Autodesk Inventor part; units mm, degrees
ref_plane "YZ Plane" through (0, 0, 0) normal (1, 0, 0) x (0, 1, 0)
ref_plane "XZ Plane" through (0, 0, 0) normal (0, 1, 0) x (-1, 0, 0)
ref_plane "XY Plane" through (0, 0, 0) normal (0, 0, 1) x (1, 0, 0)
sketch "Skizze1" plane through (0, 0, 0) normal (0, 0, 1) x (1, 0, 0)
  line L0 (-39.95, 42.95) -> (-39.95, -42.95)
  line L1 (-39.95, -42.95) -> (39.95, -42.95)
  line L2 (39.95, -42.95) -> (39.95, 42.95)
  line L3 (39.95, 42.95) -> (-39.95, 42.95)
  line L4 (-36.95, 39.95) -> (-15, 39.95)
  line L5 (36.95, 39.95) -> (36.95, -39.95)
  line L6 (36.95, -39.95) -> (-36.95, -39.95)
  line L7 (-36.95, -39.95) -> (-36.95, 39.95)
  line L8 (-36.95, 39.95) -> (36.95, -39.95) construction
  line L9 (36.95, 39.95) -> (-36.95, -39.95) construction
  line L10 (0, -67.13) -> (0, 67.13)
  line L11 (-15, 39.95) -> (-15, 42.95)
  line L12 (15, 39.95) -> (15, 42.95)
  line L13 (15, 39.95) -> (36.95, 39.95)
  line L14 (44.95, -47.95) -> (-44.95, -47.95)
  line L15 (-44.95, -47.95) -> (-44.95, 47.95)
  line L16 (-44.95, 47.95) -> (-15, 47.95)
  line L17 (44.95, 47.95) -> (44.95, -47.95)
  line L18 (44.95, -47.95) -> (-44.95, 47.95) construction
  line L19 (-44.95, -47.95) -> (44.95, 47.95) construction
  line L20 (-15, 42.95) -> (-15, 47.95)
  line L21 (15, 42.95) -> (15, 47.95)
  line L22 (15, 47.95) -> (44.95, 47.95)
  point P0 (0, 0)
  point P1 (-15, 41.45)
  dimension "d0" = 3
  dimension "d1" = 3
  dimension "d2" = 30
  dimension "d4" = 5
  dimension "d5" = 5
extrude "Extrusion1" add sketch "Skizze1" along normal blind 10 contours L3 L11 L4 L7 L6 L10 L1 L0 | L0 L1 L10 L14 L15 L16 L20 L3 | L10 L6 L5 L13 L12 L3 L2 L1 | L1 L2 L3 L21 L22 L17 L14 L10
sketch "Skizze2" plane through (0, 0, 0) normal (0, 0, -1) x (-1, 0, 0)
  line L0 (-39.95, 42.95) -> (39.95, 42.95)
  line L1 (39.95, 42.95) -> (39.95, -42.95)
  line L2 (39.95, -42.95) -> (-39.95, -42.95)
  line L3 (-39.95, -42.95) -> (-39.95, 42.95)
  line L4 (-44.95, -47.95) -> (-44.95, 47.95)
  line L5 (-44.95, 47.95) -> (-15, 47.95)
  line L6 (44.95, -47.95) -> (-44.95, -47.95)
  line L7 (44.95, 47.95) -> (44.95, -47.95)
  line L8 (15, 47.95) -> (44.95, 47.95)
  line L9 (15, 39.95) -> (15, 47.95)
  line L10 (15, 47.95) -> (44.95, 47.95)
  line L11 (15, 47.95) -> (15, 42.95)
  line L12 (15, 39.95) -> (15, 47.95)
  line L13 (15, 47.95) -> (44.95, 47.95)
  line L14 (44.95, 47.95) -> (44.95, -47.95)
  line L15 (44.95, -47.95) -> (44.95, 47.95)
  line L16 (15, 42.95) -> (39.95, 42.95)
  line L17 (39.95, 42.95) -> (39.95, -42.95)
  line L18 (39.95, -42.95) -> (-39.95, -42.95)
  line L19 (-39.95, 42.95) -> (-39.95, -42.95)
  line L20 (-39.95, 42.95) -> (-15, 42.95)
  line L21 (-15, 47.95) -> (-15, 39.95)
  line L22 (-15, 42.95) -> (-15, 47.95)
  line L23 (-44.95, -47.95) -> (-44.95, 47.95)
  line L24 (-15, 47.95) -> (-44.95, 47.95)
  line L25 (-44.95, 47.95) -> (-44.95, -47.95)
  line L26 (-40.1, -43.1) -> (40.1, -43.1)
  line L27 (40.1, -43.1) -> (40.1, 43.1)
  line L28 (40.1, 43.1) -> (-40.1, 43.1)
  line L29 (-40.1, 43.1) -> (-40.1, -43.1)
  line L30 (-40.1, -43.1) -> (40.1, 43.1) construction
  line L31 (40.1, -43.1) -> (-40.1, 43.1) construction
  point P0 (0, 0)
  point P1 (15, 43.1)
  point P2 (-15, 43.1)
  dimension "d35" = 80.2
  dimension "d36" = 86.2
extrude "Extrusion2" add sketch "Skizze2" along normal blind 1.6 contours L28 L29 L26 L27 L9 L8 L7 L6 L4 L5 L21
sketch "Skizze3" plane through (0, 0, 10) normal (0, 0, 1) x (1, 0, 0)
  line L0 (44.95, -47.95) -> (-44.95, -47.95)
  line L1 (-44.95, 47.95) -> (44.95, 47.95)
  line L2 (44.95, 47.95) -> (44.95, -47.95)
  line L3 (44.95, -47.95) -> (-44.95, -47.95)
  line L4 (-44.95, -47.95) -> (-44.95, 47.95)
  point P0 (0, 0)
extrude "Extrusion3" add sketch "Skizze3" along normal blind 2
sketch "Skizze4" plane through (0, 0, 10) normal (0, 0, -1) x (-1, 0, 0)
  line L0 (15, 39.95) -> (15, 47.95)
  line L1 (-15, 47.95) -> (15, 47.95)
  line L2 (-15, 47.95) -> (-15, 39.95)
  line L3 (-15, 39.95) -> (-36.95, 39.95)
  line L4 (-36.95, 39.95) -> (-36.95, -39.95)
  line L5 (-36.95, -39.95) -> (36.95, -39.95)
  line L6 (36.95, -39.95) -> (36.95, 39.95)
  line L7 (36.95, 39.95) -> (15, 39.95)
  line L8 (0, -67.13) -> (0, 67.13)
  line L9 (-15, 47.95) -> (15, 47.95)
  line L10 (15, 47.95) -> (7.5, 47.95)
  line L11 (7.5, 47.95) -> (7.5, 44.95)
  line L12 (7.5, 44.95) -> (15, 44.95)
  line L13 (15, 44.95) -> (15, 47.95)
  line L14 (-15, 39.95) -> (-15, 47.95)
  line L15 (15, 47.95) -> (-15, 47.95)
  line L16 (-7.5, 47.95) -> (-7.5, 44.95)
  line L17 (-7.5, 44.95) -> (-15, 44.95)
  point P0 (0, 0)
  point P1 (-7.5, 47.95)
  point P2 (-15, 44.95)
  point P3 (15, 44.95)
  point P4 (7.5, 47.95)
  point P5 (7.5, 46.45)
  point P6 (11.25, 47.95)
  dimension "d14" = 15
  dimension "d15" = 3
extrude "Extrusion4" add sketch "Skizze4" along normal up to surface (11.6 mm away) contours L12 L11 L1 L0 | L16 L17 L2 L1
fillet "Rundung1" radius 2 2 edges at (-7.5, 46.45, 10) (7.5, 46.45, 10)
fillet "Rundung2" [suppressed]
fillet "Rundung3" [suppressed]
sketch "Skizze5" plane through (0, 0, 10) normal (0, 0, -1) x (-1, 0, 0)
  circle A0 centre (-26.75, 21.7) radius 1.1
  circle A1 centre (27.25, 21.65) radius 1.1
  point P0 (0, 0)
extrude "Extrusion5" cut sketch "Skizze5" against normal through all
sketch "Skizze6" plane through (0, 0, 10) normal (0, 0, -1) x (-1, 0, 0)
  point P0 (0, 0)
sketch "Skizze7" plane through (0, 0, 10) normal (0, 0, -1) x (-1, 0, 0)
  circle A0 centre (27.25, 21.65) radius 1.1
  circle A1 centre (-26.75, 21.7) radius 1.1
  line L0 (-5.5, 44.95) -> (-5.5, 47.95)
  line L1 (-5.5, 44.95) -> (-15, 44.95)
  line L2 (-15, 44.95) -> (-15, 39.95)
  line L3 (-15, 39.95) -> (-36.95, 39.95)
  line L4 (-36.95, 39.95) -> (-36.95, -39.95)
  line L5 (-36.95, -39.95) -> (36.95, -39.95)
  line L6 (36.95, -39.95) -> (36.95, 39.95)
  line L7 (36.95, 39.95) -> (15, 39.95)
  line L8 (15, 39.95) -> (15, 44.95)
  line L9 (15, 44.95) -> (5.5, 44.95)
  line L10 (5.5, 47.95) -> (5.5, 44.95)
  circle A2 centre (27.25, 21.65) radius 1.1
  circle A3 centre (27.25, 21.65) radius 4.5
  line L11 (0, -67.13) -> (0, 67.13)
  circle A4 centre (-26.75, 21.7) radius 4.5
  line L12 (-5.5, 47.95) -> (5.5, 47.95)
  point P0 (0, 0)
  dimension "d21" = 9
extrude "Extrusion6" add sketch "Skizze7" along normal blind 9.5 contours A3 | A4
sketch "Skizze8" plane through (0, 0, 12) normal (0, 0, 1) x (1, 0, 0)
  line L0 (0, -67.13) -> (0, 67.13)
  circle A0 centre (-27.25, 21.65) radius 1.1
  circle A1 centre (-27.25, 21.65) radius 2.25
  circle A2 centre (26.75, 21.7) radius 1.1
  circle A3 centre (26.75, 21.7) radius 2.25
  point P0 (0, 0)
  dimension "d24" = 4.5
  dimension "d25" = 4.5
extrude "Extrusion7" cut sketch "Skizze8" against normal blind 10.5
chamfer "Fase1" distance 2 angle 45 4 edges at (44.95, 0, 12) (0, -47.95, 12) (0, 47.95, 12) (-44.95, 0, 12)
chamfer "Fase2" distance 2 angle 45 4 edges at (-44.95, 47.95, 4.2002) (-44.95, -47.95, 4.2003) (44.95, -47.95, 4.2003) (44.95, 47.95, 4.2002)
properties part number "Bottom" material "Glas"
Can you work these out from the model? Positions are in its coordinate system, mm. A direction names the side the tool comes from. Coordinates: 2 decimals unless noted, no trailing zeros. Write each loop counter-clockwise with the first axis right and the second up, starting at its lowest first coordinate (ties: lowest second). Pieces come first, ordered by that corner, then holes. Notation, with made-up numbers: (33.25, -14.5) -> (38.25, -14.5) arc R15 cw to (38.25, 2.5) -> close; hole circle Ø1 at (-6.75, 73.5). An arc over 180 degrees is marked (long way). Write item = value, one per line.
(1) Imagine slicing it at A-A (x = -27.25). Please give me the cut outline in (y, z), and give its area (3 significant figures).
Verdict:
outline = (-47.95, -1.6) -> (-43.1, -1.6) -> (-43.1, 0) -> (-39.95, 0) -> (-39.95, 10) -> (17.15, 10) -> (17.15, 0.5) -> (20.55, 0.5) -> (20.55, 1.5) -> (19.4, 1.5) -> (19.4, 12) -> (-45.95, 12) -> (-47.95, 10) -> close; (22.75, 0.5) -> (26.15, 0.5) -> (26.15, 10) -> (39.95, 10) -> (39.95, 0) -> (43.1, 0) -> (43.1, -1.6) -> (47.95, -1.6) -> (47.95, 10) -> (45.95, 12) -> (23.9, 12) -> (23.9, 1.5) -> (22.75, 1.5) -> close
area = 399 mm^2
(2) Thinking about a two-plate mould opening in X: for faces 6 (the face through (-44.95, -1, 4)), 7 (the face through (36.95, 1, 5)), 8 (the face through (9, 47.95, 4)), which applies, +X half, -X half, draft (parallel to the pull), parting line (faces both ways), or undercut?
Verdict:
face_6 = -X half
face_7 = undercut
face_8 = draft
(3) Imagine slicing it at C-C (x = 11.5). Please give me the cut outline in (y, z), and give its area (3 significant figures).
Verdict:
outline = (-47.95, -1.6) -> (-43.1, -1.6) -> (-43.1, 0) -> (-39.95, 0) -> (-39.95, 10) -> (44.95, 10) -> (44.95, -1.6) -> (47.95, -1.6) -> (47.95, 10) -> (45.95, 12) -> (-45.95, 12) -> (-47.95, 10) -> close
area = 310 mm^2
(4) Imagine slicing it at B-B (z = 3.5). Please give me the cut outline in (x, y).
Verdict:
outline = (-44.95, -45.95) -> (-42.95, -47.95) -> (42.95, -47.95) -> (44.95, -45.95) -> (44.95, 45.95) -> (42.95, 47.95) -> (7.5, 47.95) -> (7.5, 44.95) -> (15, 44.95) -> (15, 39.95) -> (36.95, 39.95) -> (36.95, -39.95) -> (-36.95, -39.95) -> (-36.95, 39.95) -> (-15, 39.95) -> (-15, 44.95) -> (-7.5, 44.95) -> (-7.5, 47.95) -> (-42.95, 47.95) -> (-44.95, 45.95) -> close; circle Ø9 at (-27.25, 21.65); circle Ø9 at (26.75, 21.7); hole circle Ø4.5 at (-27.25, 21.65); hole circle Ø4.5 at (26.75, 21.7)
(5) For pin 1 (0.9 mm diameter, centred on y = 47, z = 5, fed in from -X); pin 2 (1.3 mm diameter, centred on x = 26.5, y = 20.5, fed in from +Z); pin 3 (0.8 mm diameter, centred on x = -5.5, z = -1, fed in from +Y), each with a flat end and sliding along its axis, tell me the tip position at first contact or that it passes through.
Verdict:
pin_1 = -44.35
pin_2 = 1.5
pin_3 = -43.1
(6) Imagine slicing it at D-D (y = 38). Please give me the cut outline in (x, z).
Verdict:
outline = (-44.95, -1.6) -> (-40.1, -1.6) -> (-40.1, 0) -> (-36.95, 0) -> (-36.95, 10) -> (36.95, 10) -> (36.95, 0) -> (40.1, 0) -> (40.1, -1.6) -> (44.95, -1.6) -> (44.95, 10) -> (42.95, 12) -> (-42.95, 12) -> (-44.95, 10) -> close
(7) If I drill on probe 1 along Y at (x, z) = (26.75, 4.75); probe 2 along Y at (x, z) = (35, 7.75); probe 3 along Y at (x, z) = (-27.25, 1.2), over which ranges is the centre line in solid material (lowest first)?
Verdict:
probe_1 = -47.95 to -39.95, 17.2 to 19.45, 23.95 to 26.2, 39.95 to 47.95
probe_2 = -47.95 to -39.95, 39.95 to 47.95
probe_3 = -47.95 to -39.95, 17.15 to 20.55, 22.75 to 26.15, 39.95 to 47.95
(8) On a 3-axis mill with a long thin cutter (end or side, diameter ignored), from which of +Z, -Z, +X, -X, +Y, -Y can I reach the whole of each face in a straight line? I mean faces 1 (the face through (0.62, -46.96, 10.99)), 2 (the face through (43, -3, -1.6)), 3 (the face through (7.5, 46, 3)), 4 (the face through (26, 39.95, 5)), 5 (the face through (-26, 22, 1.5)). Say none if no direction works.
Verdict:
face_1 = +Z, +X, -X, -Y
face_2 = -Z, +X, -X, +Y, -Y
face_3 = -Z, +Y
face_4 = -Z
face_5 = +Z
